```python
from build123d import *

# Parameters (mm, degrees)
BOSS_EXTRUDE1_DEPTH                             = 3.175
SKETCH2_R                                       = 3.175
CUT_EXTRUDE1_DEPTH                              = 4.175
FILLET1_R                                       = 20.32
CSK_FOR_M3_FLAT_HEAD_MACHINE_SCREW1_D           = 3.4
CSK_FOR_M3_FLAT_HEAD_MACHINE_SCREW1_DEPTH       = 3.175
CSK_FOR_M3_FLAT_HEAD_MACHINE_SCREW1_CSINK_D     = 6.3
CSK_FOR_M3_FLAT_HEAD_MACHINE_SCREW1_CSINK_ANGLE = 90
F_10_0_1935_DIAMETER_HOLE1_D                    = 4.9149
F_10_0_1935_DIAMETER_HOLE1_DEPTH                = 3.175
F_10_0_1935_DIAMETER_HOLE2_D                    = 4.9149
F_10_0_1935_DIAMETER_HOLE2_DEPTH                = 3.175
F_10_0_1935_DIAMETER_HOLE3_D                    = 4.9149
F_10_0_1935_DIAMETER_HOLE3_DEPTH                = 3.175
SKETCH17_R                                      = 3.175
CUT_EXTRUDE2_DEPTH                              = 4.175


with BuildPart() as part:
    # Sketch1 → Boss-Extrude1 (new body)
    with BuildSketch(Plane(origin=(0, 0, 0), x_dir=(1, 0, 0), z_dir=(0, 1, 0))):
        with BuildLine():
            Line((36.5125, 0), (-36.5125, 0))
            Line((-36.5125, 0), (-36.5125, 63.5))
            ThreePointArc((-36.5125, 63.5), (-211.232921163, 122.820712342), (-295.17951094, 287.134870433))
            ThreePointArc((-295.17951094, 287.134870433), (-272.075392256, 314.639773629), (-244.57048906, 291.535654944))
            ThreePointArc((-244.57048906, 291.535654944), (-50.8, 113.883561638), (142.97048906, 291.535654944))
            ThreePointArc((142.97048906, 291.535654944), (170.475392256, 314.639773629), (193.57951094, 287.134870433))
            ThreePointArc((193.57951094, 287.134870433), (144.953596881, 160.556125349), (36.5125, 79.148590487))
            Line((36.5125, 79.148590487), (36.5125, 0))
        make_face()
    extrude(amount=BOSS_EXTRUDE1_DEPTH)

    # Sketch2 → Cut-Extrude1 (cut, through all)
    with BuildSketch(Plane(origin=(0, 3.175, 0), x_dir=(1, 0, 0), z_dir=(0, 1, 0))):
        with Locations((-269.875, 289.335262689)):
            Circle(SKETCH2_R)
        with Locations((168.275, 289.335262689)):
            Circle(SKETCH2_R)
    extrude(amount=-CUT_EXTRUDE1_DEPTH, mode=Mode.SUBTRACT)

    # Fillet1
    fillet1_edges = [part.edges().sort_by_distance(p)[0] for p in [
        (-36.5125, 1.5875, -63.5),
        (36.5125, 1.5875, -79.148590487),
    ]]
    fillet(fillet1_edges, radius=FILLET1_R)

    # CSK for M3 Flat Head Machine Screw1
    with Locations(Plane(origin=(0, 3.175, 0), x_dir=(1, 0, 0), z_dir=(0, 1, 0))):
        with Locations((-269.875, 305.335262689), (168.275, 305.335262689), (182.131406461, 297.335262689), (182.131406461, 281.335262689), (168.275, 273.335262689), (154.418593539, 281.335262689), (154.418593539, 297.335262689), (-256.018593539, 297.335262689), (-256.018593539, 281.335262689), (-269.875, 273.335262689), (-283.731406461, 281.335262689), (-283.731406461, 297.335262689)):
            CounterSinkHole(CSK_FOR_M3_FLAT_HEAD_MACHINE_SCREW1_D / 2, CSK_FOR_M3_FLAT_HEAD_MACHINE_SCREW1_CSINK_D / 2, depth=CSK_FOR_M3_FLAT_HEAD_MACHINE_SCREW1_DEPTH, counter_sink_angle=CSK_FOR_M3_FLAT_HEAD_MACHINE_SCREW1_CSINK_ANGLE)

    # #10 (0.1935) Diameter Hole1
    with Locations(Plane(origin=(0, 3.175, 0), x_dir=(1, 0, 0), z_dir=(0, 1, 0))):
        with Locations((-26.9875, 12.7), (-26.9875, 38.1), (0, 38.1), (0, 12.7), (26.9875, 12.7), (26.9875, 38.1)):
            Hole(F_10_0_1935_DIAMETER_HOLE1_D / 2, depth=F_10_0_1935_DIAMETER_HOLE1_DEPTH)

    # #10 (0.1935) Diameter Hole2
    with Locations(Plane(origin=(0, 3.175, 0), x_dir=(1, 0, 0), z_dir=(0, 1, 0))):
        with Locations((87.3125, 117.294734137), (108.272403388, 136.716708161), (129.232306776, 156.138682184), (-188.9125, 117.294734137), (-209.872403388, 136.716708161), (-230.832306776, 156.138682184)):
            Hole(F_10_0_1935_DIAMETER_HOLE2_D / 2, depth=F_10_0_1935_DIAMETER_HOLE2_DEPTH)

    # #10 (0.1935) Diameter Hole3
    with Locations(Plane(origin=(0, 3.175, 0), x_dir=(1, 0, 0), z_dir=(0, 1, 0))):
        with Locations((-63.5, 98.392247698), (44.141179096, 120.65), (138.157224076, 215.9), (-239.757224076, 215.9), (-145.741179096, 120.65)):
            Hole(F_10_0_1935_DIAMETER_HOLE3_D / 2, depth=F_10_0_1935_DIAMETER_HOLE3_DEPTH)

    # Sketch17 → Cut-Extrude2 (cut, through all)
    with BuildSketch(Plane(origin=(0, 3.175, 0), x_dir=(1, 0, 0), z_dir=(0, 1, 0))):
        with Locations((-26.9875, 25.4)):
            Circle(SKETCH17_R)
        with Locations((0, 25.4)):
            Circle(SKETCH17_R)
        with Locations((26.9875, 25.4)):
            Circle(SKETCH17_R)
    extrude(amount=-CUT_EXTRUDE2_DEPTH, mode=Mode.SUBTRACT)


solid = part.part
```
Part model, mm, in its own coordinate system. Round coordinates to 2 decimals unless told otherwise and drop trailing zeros. Write each loop counter-clockwise with the first axis right and the second up, starting at its lowest first coordinate (ties: lowest second). Pieces come first, ordered by that corner, then holes. Notation, with made-up numbers: (16, -1.5) -> (69, -1.5) arc R10 ccw to (69, 15.5) -> close; hole circle Ø11 at (-19, -20.75). An arc over 180 degrees is marked (long way). Return JSON: item names as keys, results as strings. Group by question number.
Q1. Pin check, flat tips, straight feed: pin 1 (1.5 mm diameter, centred on x = 86, y = 2.5, fed in from +Z); pin 2 (1.5 mm diameter, centred on y = 2, z = -95.5, fed in from -X); pin 3 (1 mm diameter, centred on y = 1, z = -21, fed in from -X). Stop position of each tip, or through.
Q2. Saw through at D-D on z = -148. Write the cut outline in (x, y) (3 decimals), plus the area to 3 significant figures.
Q3. Saw through at C-C on y = 0.5. State how many separate pieces and enclosed holes the cut face has, plus the area to 3 significant figures.
Q4. Saw through at A-A on z = -263. Write the cut outline in (x, y) (3 decimals).
Q5. Saw through at B-B on x = -13.5. Write the cut outline in (y, z) (3 decimals), plus the area to 3 significant figures.
Q6. Mould opens along X. For faces 1 (the cylindrical face through (-42.15, 1.61, -56.88)), 2 (the cylindrical face through (169.92, 1.57, -314.68)), 3 (the flat face through (-68, 3.175, -111)), 4 (the cylindrical face through (-54.841, 1.565, -113.926)) say: pulls with the +X half, pulls with the -X half, needs draft (parallel to the pull), parting line crosses it, or undercut.
Q7. Probe L1, parallel to X at y = 1.1, z = -215.9; L2, parallel to Z at x = -269, y = 3.05; L3, parallel to Z at x = 0, y = 1 (3 decimals). List the from-to ranges inside material, lowest first. Write a range as [from, to].
Answer:
{
 "1": {"pin 1": "z = -104.27", "pin 2": "x = -173.97", "pin 3": "x = -36.51"},
 "2": {"outline": "(-236.406, 0) -> (-160.834, 0) -> (-160.834, 3.175) -> (-236.406, 3.175) -> close; (59.234, 0) -> (134.806, 0) -> (134.806, 3.175) -> (59.234, 3.175) -> close", "area": "480 mm2"},
 "3": {"separate pieces": "1", "enclosed holes": "34", "area": "39,800 mm2"},
 "4": {"outline": "(-291.867, 0) -> (-239.932, 0) -> (-239.932, 3.175) -> (-291.867, 3.175) -> close; (138.332, 0) -> (190.267, 0) -> (190.267, 3.175) -> (138.332, 3.175) -> close"},
 "5": {"outline": "(0, -117.494) -> (3.175, -117.494) -> (3.175, 0) -> (0, 0) -> close", "area": "373 mm2"},
 "6": {"face 1": "pulls with the -X half", "face 2": "undercut", "face 3": "needs draft", "face 4": "undercut"},
 "7": {"L1": "[-278, -242.21], [-237.3, -221.91], [120.31, 135.7], [140.61, 176.4]", "L2": "[-314.72, -308.23], [-302.44, -292.39], [-286.28, -276.23], [-270.44, -196.31]", "L3": "[-120.635, -40.557], [-35.643, -28.575], [-22.225, -15.157], [-10.243, 0]"}
}
